The listing builds one solid part. Answer for the finished solid, in the listing's coordinates (mm). Face numbers are marked on the shaded views. A direction names the side the tool comes from. Give positions to 0.01 mm unless a question says otherwise; leave off trailing zeros. Order: outer loops, then holes, each group sorted by start corner. A loop starts at its lowest first (then second) coordinate and runs counter-clockwise, first axis right, second up. Notation, with made-up numbers: (-20.75, 10) - (-13.75, 10) arc R34 cw to (-13.75, 41) - close; hole circle Ø3 at (38, 59). An arc over 180 degrees is marked (long way). Use a Markdown table: item, result. Add a question column.
1) Find section A-A, the plane z = 203. Determine the outline of the cut face in (x, y).
2) Find section C-C, the plane y = -86.5. Determine the outline of the cut face in (x, z), plus the area to 3 significant figures.
3) Find section D-D, the plane z = 127. Determine the outline of the cut face in (x, y).
4) Straight lines are drawn through the part: line 1 (Y direction, x = 66, z = 117); line 2 (Z direction, x = 374, y = 21); line 3 (Z direction, x = 56, y = -126.5). For each, find the intervals that lie inside material, in ascending order.
5) Flat-ended cylindrical pins translate along their axes: pin 1 (2 mm diameter, centred on x = 130.5, z = 111.5, fed in from -Y); pin 2 (23 mm diameter, centred on x = 244.5, z = 131, fed in from +Y); pin 3 (23 mm diameter, centred on y = -15, z = 199, fed in from -X). Find the tip coordinate at first contact, or state that the pin passes through.
6) Find section B-B, the plane x = 91.5. Determine the outline of the cut face in (y, z), plus the area to 3 significant figures.
7) For the marked faces 1, 2, 3, 4 and 5, determine the directions among +Z, -Z, +X, -X, +Y, -Y from which every point of the face is accessible in a straight line to the end or side of a thin tool.
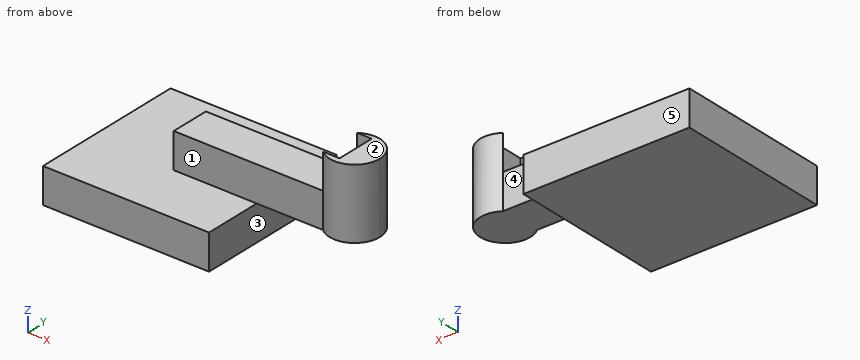
from build123d import *

# Parameters (mm, degrees)
F0_W     = 361.632824
F0_H     = 342.431128
F2_DEPTH = 76.2
F1_W     = 361.180782
F1_H     = 86.339838
F3_DEPTH = 152.4
F5_DEPTH = 76.2
F6_W     = 180.36437
F6_H     = 76.2
F7_DEPTH = 214.386483


with BuildPart() as f2:
    # F0 (on Top) → F2 (new body)
    with BuildSketch(Plane.XY):
        Rectangle(F0_W, F0_H)
    extrude(amount=F2_DEPTH)

    # F1 (on Top) → F3 (join)
    with BuildSketch(Plane.XY):
        with Locations((180.590391, 0)):
            Rectangle(F1_W, F1_H)
    extrude(amount=F3_DEPTH)

    # F4 (on face) → F5 (join, symmetric)
    with BuildSketch(Plane.XY.offset(152.4)):
        with BuildLine():
            ThreePointArc((325.230616, -43.169919), (383.41811, -51.064962), (415.034036, -1.582143))
            ThreePointArc((415.034036, -1.582143), (385.746466, 46.754361), (329.343175, 43.169919))
            Line((329.343175, 43.169919), (361.180782, 43.169919))
            Line((361.180782, 43.169919), (361.180782, -43.169919))
            Line((361.180782, -43.169919), (325.230616, -43.169919))
        make_face()
    extrude(amount=F5_DEPTH, both=True)

    # F6 (on face) → F7 (cut, through all)
    with BuildSketch(Plane(origin=(0, 43.169919, 0), x_dir=(-1, 0, 0), z_dir=(0, 1, 0))):
        with Locations((-270.998597, 38.1)):
            Rectangle(F6_W, F6_H)
    extrude(amount=-F7_DEPTH, mode=Mode.SUBTRACT)


solid = f2.part
The answers:
| question | item | result |
|---|---|---|
| 1 | outline | (325.23, -43.17) arc R54.53 ccw (long way) to (329.34, 43.17) - (361.18, 43.17) - (361.18, -43.17) - close |
| 2 | outline | (-180.82, 0) - (180.82, 0) - (180.82, 76.2) - (-180.82, 76.2) - close |
| 2 | area | 27,600 mm2 |
| 3 | outline | (0, -43.17) - (325.23, -43.17) arc R54.53 ccw (long way) to (329.34, 43.17) - (0, 43.17) - close |
| 4 | line 1 | -43.17 to 43.17 |
| 4 | line 2 | 76.2 to 228.6 |
| 4 | line 3 | 0 to 76.2 |
| 5 | pin 1 | y = -43.17 |
| 5 | pin 2 | y = 43.17 |
| 5 | pin 3 | x = 361.18 |
| 6 | outline | (-171.22, 0) - (171.22, 0) - (171.22, 76.2) - (43.17, 76.2) - (43.17, 152.4) - (-43.17, 152.4) - (-43.17, 76.2) - (-171.22, 76.2) - close |
| 6 | area | 32,700 mm2 |
| 7 | face 1 | +Z, -X, -Y |
| 7 | face 2 | +Z, +X, -X, +Y, -Y |
| 7 | face 3 | -Z, +X, +Y, -Y |
| 7 | face 4 | +Z, -X, +Y |
| 7 | face 5 | +Z, -Z, +X, -X, +Y |
